Verification items for the finished model (mm, model axes). A direction names the side the tool comes from. Round coordinates to 2 decimals unless told otherwise and drop trailing zeros. Write each loop counter-clockwise with the first axis right and the second up, starting at its lowest first coordinate (ties: lowest second). Pieces come first, ordered by that corner, then holes. Notation, with made-up numbers: (27.5, 29.5) - (66.5, 29.5) arc R28 cw to (66.5, 48.5) - close; hole circle Ø3 at (6.25, -39.5). An arc over 180 degrees is marked (long way). Answer as a JSON object with one key per item and string values.
```python
from build123d import *

# Parameters (mm, degrees)
ESQUISSE1_W        = 20
ESQUISSE1_H        = 5
ESQUISSE1_W_2      = 40
ESQUISSE1_H_2      = 20
ESQUISSE1_W_3      = 30
BOSS_EXTRU_1_DEPTH = 5


with BuildPart() as part:
    # Esquisse1 → Boss.-Extru.1 (new body)
    with BuildSketch(Plane.XY):
        Polygon((-100, 150), (100, 150), (100, 90), (105, 90), (105, 150), (113, 150), (113, 0), (-113, 0), (-113, 150), (-105, 150), (-105, 90), (-100, 90), align=None)
        with Locations((90, 7.5)):
            Rectangle(ESQUISSE1_W, ESQUISSE1_H, mode=Mode.SUBTRACT)
        with Locations((90, 77.5)):
            Rectangle(ESQUISSE1_W, ESQUISSE1_H, mode=Mode.SUBTRACT)
        Polygon((-15, 5), (15, 5), (15, 10), (0, 10), (-15, 10), align=None, mode=Mode.SUBTRACT)
        Polygon((-15, 80), (0, 80), (15, 80), (15, 75), (-15, 75), align=None, mode=Mode.SUBTRACT)
        with Locations((-90, 7.5)):
            Rectangle(ESQUISSE1_W, ESQUISSE1_H, mode=Mode.SUBTRACT)
        with Locations((-90, 77.5)):
            Rectangle(ESQUISSE1_W, ESQUISSE1_H, mode=Mode.SUBTRACT)
        with Locations((45, 25)):
            Rectangle(ESQUISSE1_W_2, ESQUISSE1_H_2, mode=Mode.SUBTRACT)
        with Locations((70, 132.5)):
            Rectangle(ESQUISSE1_W_3, ESQUISSE1_H, mode=Mode.SUBTRACT)
    extrude(amount=BOSS_EXTRU_1_DEPTH)


solid = part.part
```
Q1. Material ranges on line 1 along X through (y, z) = (97, 3.8); line 2 along Y through (x, z) = (-86.5, 4.8); line 3 along X through (y, z) = (130.5, 4.5), recorded low to high. Write a range as [from, to].
Geometry check:
{"line 1": "x = [-113, -105], [-100, 100], [105, 113]", "line 2": "y = [0, 5], [10, 75], [80, 150]", "line 3": "x = [-113, -105], [-100, 55], [85, 100], [105, 113]"}
Q2. Section check D-D, the plane z = 2.5. State how many separate pieces and enclosed holes the cut face has, then the cut area to 4 significant figures.
Geometry check:
{"separate pieces": "1", "enclosed holes": "8", "area": "31,650 mm2"}
Q3. Section check C-C, the plane y = 104.5. Record the cut outline in (x, z).
Geometry check:
{"outline": "(-113, 0) - (-105, 0) - (-105, 5) - (-113, 5) - close; (-100, 0) - (100, 0) - (100, 5) - (-100, 5) - close; (105, 0) - (113, 0) - (113, 5) - (105, 5) - close"}
Q4. Section check B-B, the plane y = 19. Record the cut outline in (x, z).
Geometry check:
{"outline": "(-113, 0) - (25, 0) - (25, 5) - (-113, 5) - close; (65, 0) - (113, 0) - (113, 5) - (65, 5) - close"}
Q5. Section check A-A, the plane x = 9.5. Record the cut outline in (y, z), then the cut area to 3 significant figures.
Geometry check:
{"outline": "(0, 0) - (5, 0) - (5, 5) - (0, 5) - close; (10, 0) - (75, 0) - (75, 5) - (10, 5) - close; (80, 0) - (150, 0) - (150, 5) - (80, 5) - close", "area": "700 mm2"}
Q6. Gauge pin test, flat ends, axial feed: P1, Ø10, axis at x = 1.5, y = 15.5, coming from the -Z side; P2, Ø2.5, axis at x = 103.5, z = 3.5, coming from the +Y side. Record the tip position at first contact, or that the pin passes through.
Geometry check:
{"P1": "stops at z = 0", "P2": "stops at y = 90"}
Q7. Set-up check for faces 1 (the flat face through (2, 93, 5)), 2 (the flat face through (0, 75, 2)), 3 (the flat face through (102, 90, 2)): record each of +Z, -Z, +X, -X, +Y, -Y from which the full face is reachable in a straight line by a thin tool's end or side.
Geometry check:
{"face 1": "+Z, +X, -X, +Y, -Y", "face 2": "+Z, -Z", "face 3": "+Z, -Z, +Y"}
